from build123d import *

# Parameters (mm, degrees)
F0_R     = 33.75
F1_DEPTH = 72.4
F2_R     = 8


with BuildPart() as f1:
    # F0 (on Top) → F1 (new body)
    with BuildSketch(Plane.XY):
        Polygon((0, -69.282032), (60, -34.641016), (60, 34.641016), (0, 69.282032), (-60, 34.641016), (-60, -34.641016), align=None)
        Circle(F0_R, mode=Mode.SUBTRACT)
        Polygon((60, 34.641016), (60, -34.641016), (120, -69.282032), (180, -34.641016), (180, 34.641016), (120, 69.282032), align=None)
        with Locations((120, 0)):
            Circle(F0_R, mode=Mode.SUBTRACT)
        Polygon((180, 34.641016), (180, -34.641016), (240, -69.282032), (300, -34.641016), (300, 34.641016), (240, 69.282032), align=None)
        with Locations((240, 0)):
            Circle(F0_R, mode=Mode.SUBTRACT)
    extrude(amount=F1_DEPTH)

    # F2
    f2_edges = [f1.edges().sort_by_distance(p)[0] for p in [
        (60, -34.641016, 36.2),
        (0, -69.282032, 36.2),
        (-60, -34.641016, 36.2),
        (120, -69.282032, 36.2),
        (180, -34.641016, 36.2),
        (180, 34.641016, 36.2),
        (120, 69.282032, 36.2),
        (0, 69.282032, 36.2),
        (60, 34.641016, 36.2),
        (-60, 34.641016, 36.2),
        (240, -69.282032, 36.2),
        (300, -34.641016, 36.2),
        (300, 34.641016, 36.2),
        (240, 69.282032, 36.2),
    ]]
    fillet(f2_edges, radius=F2_R)


solid = f1.part
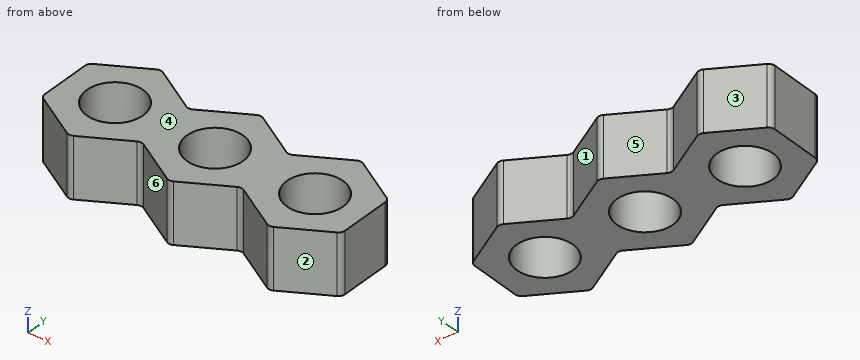
Input: part model. Units: mm. Frame: model coordinates. Face numbers are marked on the shaded views. A direction names the side the tool comes from. Coordinates: 2 decimals unless noted, no trailing zeros. Loops run counter-clockwise (first coordinate to the right, second up) from the corner with the lowest first, then second, coordinate; pieces in that order, holes last. Notation, with made-up numbers: (86, 1.25) -> (94, 1.25) arc R27 cw to (94, 19.25) -> close; hole circle Ø6 at (52.5, -9). An arc over 180 degrees is marked (long way). Write each question's results on one line, items separated by ' | '. Start each with the question number.
Q1. Reachability of the marked faces 4, 5 and 6 from +Z, -Z, +X, -X, +Y, -Y: full face, straight path, thin tool, end or side. Return the list, or none.
Q2. Section C-C, the plane y = 42. Return the cut outline in (x, z).
Q3. Pull-direction query (X, two-part tool) for the marked faces 1, 2 and 3; classes: released by +X, released by -X, zero draft, split by the parting line, or undercut.
Q4. Section B-B, the plane x = 120. Return the cut outline in (y, z).
Q5. Ray query, line 1 (X direction, y = 47, z = 42); line 2 (X direction, y = -57.5, z = 69); line 3 (X direction, y = -24, z = 23). Return the intervals inside material, ascending. Write a range as from..to.
Q6. Section D-D, the plane z = 58.5. State how many separate pieces and enclosed holes the cut face has, plus the area to 3 significant figures.
Q7. Pin query (flat end, axial travel): pin 1 (8 mm diameter, centred on x = 178.5, z = 13, fed in from -Y); pin 2 (5 mm diameter, centred on x = 4, z = 35.5, fed in from +Y); pin 3 (10 mm diameter, centred on x = 211.5, z = 24.5, fed in from +Y); pin 4 (1.5 mm diameter, centred on x = 150, y = -35, fed in from -Z). Return the tip coordinate at first contact, or that it passes through.
Q8. Section A-A, the plane y = 0. Return the cut outline in (x, z), plus the area to 3 significant figures.
Found:
1) face 4: +Z, +X, -X, +Y, -Y | face 5: +Z, -Z, +Y | face 6: +Z, -Z, -Y
2) outline: (-47.25, 0) -> (47.25, 0) -> (47.25, 72.4) -> (-47.25, 72.4) -> close; (72.75, 0) -> (167.25, 0) -> (167.25, 72.4) -> (72.75, 72.4) -> close; (192.75, 0) -> (287.25, 0) -> (287.25, 72.4) -> (192.75, 72.4) -> close
3) face 1: undercut | face 2: released by +X | face 3: released by -X
4) outline: (-68.04, 0) -> (-33.75, 0) -> (-33.75, 72.4) -> (-68.04, 72.4) -> close; (33.75, 0) -> (68.04, 0) -> (68.04, 72.4) -> (33.75, 72.4) -> close
5) line 1: -38.59..38.59, 81.41..158.59, 201.41..278.59 | line 2: -20.41..20.41, 99.59..140.41, 219.59..260.41 | line 3: -60..-23.73, 23.73..96.27, 143.73..216.27, 263.73..300
6) separate pieces: 1 | enclosed holes: 3 | area: 26,700 mm2
7) pin 1: y = -37.82 | pin 2: y = 67.9 | pin 3: y = 55.71 | pin 4: z = 0
8) outline: (-60, 0) -> (-33.75, 0) -> (-33.75, 72.4) -> (-60, 72.4) -> close; (33.75, 0) -> (86.25, 0) -> (86.25, 72.4) -> (33.75, 72.4) -> close; (153.75, 0) -> (206.25, 0) -> (206.25, 72.4) -> (153.75, 72.4) -> close; (273.75, 0) -> (300, 0) -> (300, 72.4) -> (273.75, 72.4) -> close | area: 11,400 mm2
